```python
from build123d import *

# Parameters (mm, degrees)
F0_W      = 116.5608018637
F0_H      = 30.3723793477
F1_DEPTH  = 70.4
F2_R      = 21.7279220614
F3_R      = 20.7029342891
F4_DEPTH  = 12.9
F5_R      = 17.1540446216
F6_DEPTH  = 11.3
F7_R      = 13.170324084
F8_DEPTH  = 6.4
F9_R      = 10.5563367541
F10_DEPTH = 5
F11_R     = 8.3829862068
F12_DEPTH = 4.2
F13_W     = 12.9023790359
F13_H     = 4.7707334161
F14_DEPTH = 6.7
F15_W     = 13.5998092592
F15_H     = 4.6233572066
F16_DEPTH = 10
F17_W     = 12.6895718277
F17_H     = 4.1054487228
F18_DEPTH = 6.5
F19_R     = 6.9841097136
F20_DEPTH = 5
F21_R     = 4.8457343359
F22_DEPTH = 39.6


with BuildPart() as f1:
    # F0 (on Top) → F1 (new body)
    with BuildSketch(Plane.XY):
        with Locations((-58.2804009318, 15.1861896738)):
            Rectangle(F0_W, F0_H)
    extrude(amount=F1_DEPTH)

    # F2
    f2_edges = [f1.edges().sort_by_distance(p)[0] for p in [
        (-116.560802, 15.18619, 70.4),
        (0, 15.18619, 70.4),
        (-116.560802, 15.18619, 0),
        (0, 15.18619, 0),
    ]]
    fillet(f2_edges, radius=F2_R)

    # F3 (on face) → F4 (join)
    with BuildSketch(Plane.XZ):
        with Locations((-26.7519634217, 44.41351071)):
            Circle(F3_R)
    extrude(amount=F4_DEPTH)

    # F5 (on face) → F6 (join)
    with BuildSketch(Plane.XZ.offset(12.9)):
        with Locations((-26.7519634217, 44.41351071)):
            Circle(F5_R)
    extrude(amount=F6_DEPTH)

    # F7 (on face) → F8 (join)
    with BuildSketch(Plane.XZ.offset(24.2)):
        with Locations((-26.7519634217, 44.41351071)):
            Circle(F7_R)
    extrude(amount=F8_DEPTH)

    # F9 (on face) → F10 (join)
    with BuildSketch(Plane.XZ.offset(30.6)):
        with Locations((-26.7519634217, 44.41351071)):
            Circle(F9_R)
    extrude(amount=F10_DEPTH)

    # F11 (on face) → F12 (join)
    with BuildSketch(Plane.XZ.offset(35.6)):
        with Locations((-26.7519634217, 44.41351071)):
            Circle(F11_R)
    extrude(amount=F12_DEPTH)

    # F13 (on face) → F14 (join)
    with BuildSketch(Plane.XZ):
        with Locations((-53.0363544822, 61.6516061127)):
            Rectangle(F13_W, F13_H)
    extrude(amount=-F14_DEPTH)

    # F15 (on face) → F16 (join)
    with BuildSketch(Plane.XZ):
        with Locations((-61.4054668695, 60.4561474174)):
            Rectangle(F15_W, F15_H)
    extrude(amount=-F16_DEPTH)

    # F17 (on face) → F18 (cut)
    with BuildSketch(Plane.XZ):
        with Locations((-68.1796912104, 62.7014264464)):
            Rectangle(F17_W, F17_H)
    extrude(amount=-F18_DEPTH, mode=Mode.SUBTRACT)

    # F19 (on face) → F20 (join)
    with BuildSketch(Plane.XY.offset(70.4)):
        with Locations((-31.61893785, 15.1796527207)):
            Circle(F19_R)
    extrude(amount=F20_DEPTH)

    # F21 (on face) → F22 (cut)
    with BuildSketch(Plane.XZ.offset(39.8)):
        with Locations((-26.7519634217, 44.41351071)):
            Circle(F21_R)
    extrude(amount=-F22_DEPTH, mode=Mode.SUBTRACT)


solid = f1.part
```
Design review of the part built by this model. Coordinates are the model's own, in mm. A direction names the side the tool comes from. Give positions to 0.01 mm unless a question says otherwise; leave off trailing zeros. Write each loop counter-clockwise with the first axis right and the second up, starting at its lowest first coordinate (ties: lowest second). Pieces come first, ordered by that corner, then holes. Notation, with made-up numbers: (54, 83) -> (84, 83) arc R23 cw to (84, 109) -> close; hole circle Ø7 at (4, 12.5). An arc over 180 degrees is marked (long way). Answer in a Markdown table with one row per item.
(1) Consider section B-B (x = -33). State the section outline as (y, z) points.
Results:
| item | result |
|---|---|
| outline | (-39.8, 38.82) -> (-35.6, 38.82) -> (-35.6, 35.9) -> (-30.6, 35.9) -> (-30.6, 32.82) -> (-24.2, 32.82) -> (-24.2, 28.44) -> (-12.9, 28.44) -> (-12.9, 24.68) -> (0, 24.68) -> (0, 0) -> (30.37, 0) -> (30.37, 70.4) -> (22.03, 70.4) -> (22.03, 75.4) -> (8.33, 75.4) -> (8.33, 70.4) -> (0, 70.4) -> (0, 64.15) -> (-12.9, 64.15) -> (-12.9, 60.39) -> (-24.2, 60.39) -> (-24.2, 56.01) -> (-30.6, 56.01) -> (-30.6, 52.92) -> (-35.6, 52.92) -> (-35.6, 50) -> (-39.8, 50) -> close |
(2) To check wall thickness, follow probe 1 along Y at (x, z) = (-54, 26); probe 2 along X at (y, z) = (-14, 44.5); probe 3 along Z at (x, y) = (-22.5, 24). State the ranges of each line that lie inside material, in increasing order.
Results:
| item | result |
|---|---|
| probe 1 | 0 to 30.37 |
| probe 2 | -43.91 to -31.6, -21.91 to -9.6 |
| probe 3 | 0 to 70.4 |
(3) Consider section C-C (y = -10.5). State the section outline as (x, z) points, then the cut area to 3 significant figures.
Results:
| item | result |
|---|---|
| outline | circle Ø41.41 at (-26.75, 44.41); hole circle Ø9.69 at (-26.75, 44.41) |
| area | 1,270 mm2 |
(4) Clearance check with flat-ended pins moving along their axes: pin 1 (5 mm diameter, centred on x = -30.5, y = -12, fed in from +Z); pin 2 (8 mm diameter, centred on x = -26.75, z = 44.41, fed in from -Y); pin 3 (15 mm diameter, centred on x = -67, y = 16, fed in from +Z). State where each tip first meets the part, or that it passes through.
Results:
| item | result |
|---|---|
| pin 1 | z = 65.08 |
| pin 2 | y = -0.2 |
| pin 3 | z = 70.4 |
(5) Consider section D-D (z = 11.5). State the section outline as (x, y) points.
Results:
| item | result |
|---|---|
| outline | (-114, 0) -> (-2.56, 0) -> (-2.56, 30.37) -> (-114, 30.37) -> close |
(6) For faces 1 (the cylindrical face through (-110.36, 15.4, 63.87)), 2 (the cylindrical face through (-38.596, 15.487, 72.865)), 3 (the flat face through (-61.835, 3, 63)), list the 3-axis set-ups (+Z, -Z, +X, -X, +Y, -Y) from which the entire face can be reached by the end or side of a thin tool; tool diameter is ignored.
Results:
| item | result |
|---|---|
| face 1 | +Z, -X, +Y, -Y |
| face 2 | +Z |
| face 3 | -Y |
(7) Mouldability with a two-part tool opening along X and no side actions: class faces 4 (the flat face through (-59, 15, 70.4)), 5 (the flat face through (0, 15, 35)), 6 (the cylindrical face through (-27.843, -37.671, 52.725)), 7 (the flat face through (-68, 6.5, 63)) as +X half, -X half, draft (parallel to the pull), parting line (faces both ways), or undercut.
Results:
| item | result |
|---|---|
| face 4 | draft |
| face 5 | +X half |
| face 6 | parting line |
| face 7 | undercut |
(8) Consider section A-A (y = 17.5). State the section outline as (x, z) points.
Results:
| item | result |
|---|---|
| outline | (-116.56, 21.73) arc R21.73 ccw to (-94.83, 0) -> (-21.73, 0) arc R21.73 ccw to (0, 21.73) -> (0, 48.67) arc R21.73 ccw to (-21.73, 70.4) -> (-25.03, 70.4) -> (-25.03, 75.4) -> (-38.21, 75.4) -> (-38.21, 70.4) -> (-94.83, 70.4) arc R21.73 ccw to (-116.56, 48.67) -> close |
